Geometry check sheet. Reference: drawing and pictorial views, mm from the part's lowest x, y, z. A direction names the side the tool comes from. Round coordinates to 2 decimals unless told otherwise and drop trailing zeros. Order: outer loops, then holes, each group sorted by start corner. A loop starts at its lowest first (then second) coordinate and runs counter-clockwise, first axis right, second up. Notation, with made-up numbers: (69.25, 83.5) -> (91.25, 83.5) arc R34 cw to (91.25, 118.5) -> close; hole circle Ø5 at (9.5, 66). An arc over 180 degrees is marked (long way). Return JSON: item names as keys, results as strings. Group by question number.
1) Section check C-C on y = 0.5. State how many separate pieces and enclosed holes the cut face has, plus the area to 3 significant figures.
2) Draft check along Z on the marked faces 3 and 4. Enter one of: pulls with the +Z half, pulls with the -Z half, needs draft (parallel to the pull), parting line crosses it, or undercut.
3) Section check D-D on z = 5. Enter the section's corners in (x, y), plus the area to 3 significant figures.
4) Tool access check on the marked faces 1 and 2. Record the directions out of +Z, -Z, +X, -X, +Y, -Y that give a thin tool (end or side, any length) a straight path to the whole face; none if there is none.
5) Scan lines: L1, parallel to X at y = 0.5, z = 5.25; L2, parallel to Z at x = 0.3, y = 0.5; L3, parallel to Z at x = 4.3, y = 1.35. Record each from-to range of solid material in increasing order.
6) Depth check by flat-ended pin: pin 1 (0.6 mm diameter, centred on x = 3, y = 0.5, fed in from -Z); pin 2 (0.6 mm diameter, centred on x = 4.5, y = 0.5, fed in from +Z); pin 3 (2 mm diameter, centred on x = 2, z = 2.5, fed in from -Y). Enter the tip coordinate at first touch or a pass-through.
7) Section check B-B on x = 4.4. Enter the section's corners in (y, z).
8) Section check A-A on z = 0.5. Enter the section's corners in (x, y).
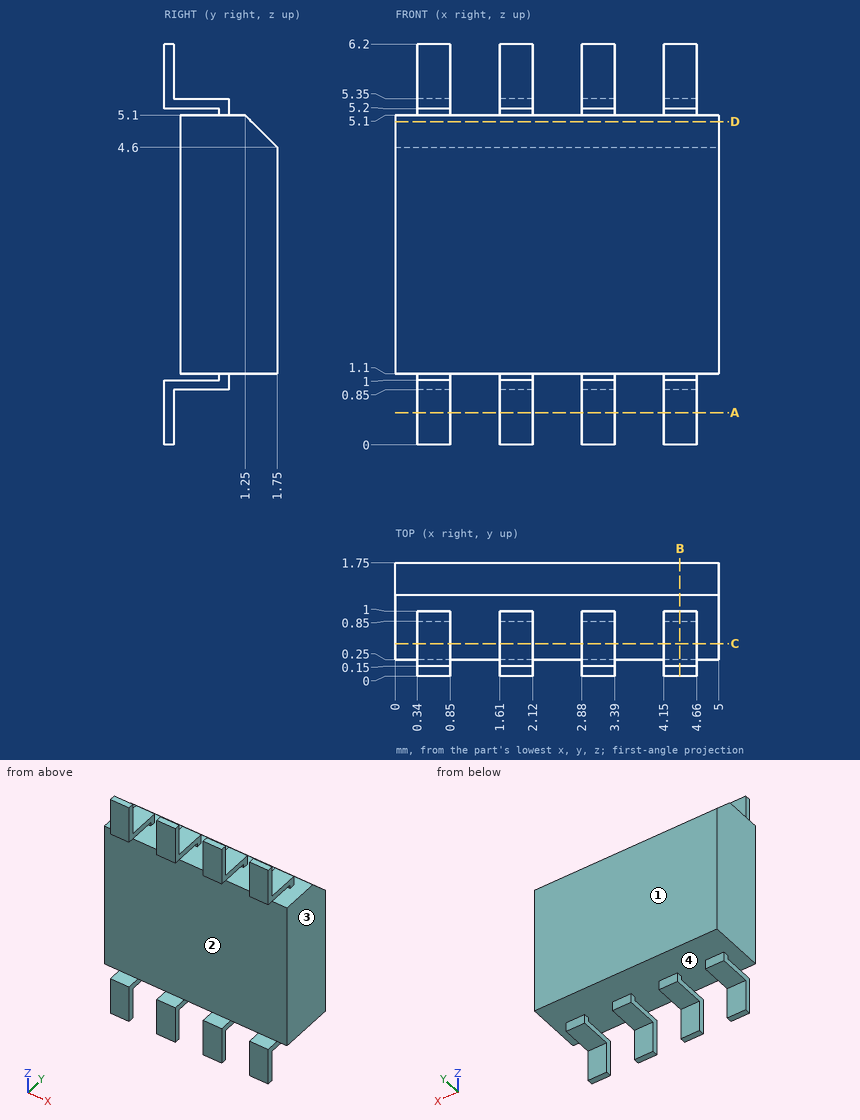
Check result:
{
 "1": {"separate pieces": "9", "enclosed holes": "0", "area": "20.6 mm^2"},
 "2": {"face 3": "needs draft", "face 4": "undercut"},
 "3": {"outline": "(0, 0.25) -> (5, 0.25) -> (5, 1.35) -> (0, 1.35) -> close", "area": "5.50 mm^2"},
 "4": {"face 1": "+Z, -Z, +X, -X, +Y", "face 2": "+X, -X, -Y"},
 "5": {"L1": "0.34 to 0.85, 1.61 to 2.12, 2.88 to 3.39, 4.15 to 4.66", "L2": "1.1 to 5.1", "L3": "1.1 to 5"},
 "6": {"pin 1": "z = 0.85", "pin 2": "z = 5.35", "pin 3": "y = 0.25"},
 "7": {"outline": "(0, 0) -> (0.15, 0) -> (0.15, 0.85) -> (1, 0.85) -> (1, 1.1) -> (1.75, 1.1) -> (1.75, 4.6) -> (1.25, 5.1) -> (1, 5.1) -> (1, 5.35) -> (0.15, 5.35) -> (0.15, 6.2) -> (0, 6.2) -> (0, 5.2) -> (0.85, 5.2) -> (0.85, 5.1) -> (0.25, 5.1) -> (0.25, 1.1) -> (0.85, 1.1) -> (0.85, 1) -> (0, 1) -> close"},
 "8": {"outline": "(0.34, 0) -> (0.85, 0) -> (0.85, 0.15) -> (0.34, 0.15) -> close; (1.61, 0) -> (2.12, 0) -> (2.12, 0.15) -> (1.61, 0.15) -> close; (2.88, 0) -> (3.39, 0) -> (3.39, 0.15) -> (2.88, 0.15) -> close; (4.15, 0) -> (4.66, 0) -> (4.66, 0.15) -> (4.15, 0.15) -> close"}
}
